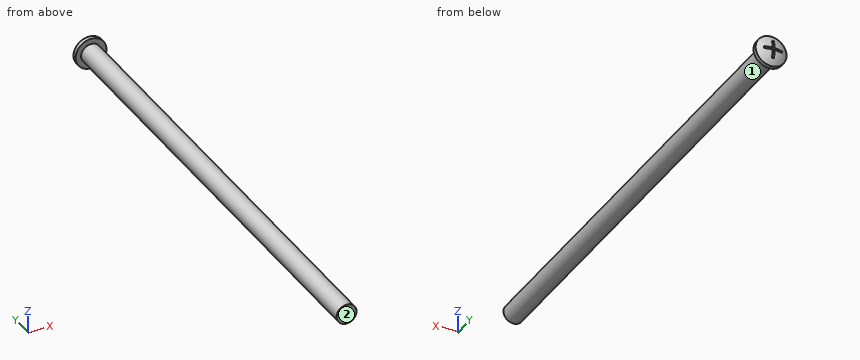
from build123d import *

# Parameters (mm, degrees)
CUT_EXTRUDE_2_DEPTH = 10


with BuildPart() as part:
    # 草图5 → 旋转1 (revolve)
    with BuildSketch(Plane.XY, mode=Mode.PRIVATE) as revolve_1_sk:
        with BuildLine():
            Line((0, -14), (-1, -14))
            Line((-1, -14), (-1, 35))
            Line((-1, 35), (-1.55, 35))
            Line((-1.55, 35), (-1.55, 35.411529967))
            add(Edge.make_bspline(
                [(-1.55, 35.411529967), (-0.860800082, 35.895988097), (0, 35.897418779)],
                knots=[0, 0, 0, 1, 1, 1], degree=2))
            Line((0, 35.897418779), (0, -14))
        make_face()
    revolve(revolve_1_sk.sketch.rotate(Axis((0, 0, 0), (0, 1, 0)), 270), axis=Axis((0, 0, 0), (0, 1, 0)))

    # 草图6 → 切除-拉伸2 (cut)
    with BuildSketch(Plane(origin=(0, 35.411529967, 0), x_dir=(-1, 0, 0), z_dir=(0, -1, 0))):
        Polygon((0.1, -0.1), (0.9, -0.1), (0.9, 0.1), (0.1, 0.1), (0.1, 0.9), (-0.1, 0.9), (-0.1, 0.1), (-0.9, 0.1), (-0.9, -0.1), (-0.1, -0.1), (-0.1, -0.9), (0.1, -0.9), align=None)
    extrude(amount=-CUT_EXTRUDE_2_DEPTH, mode=Mode.SUBTRACT)


solid = part.part
The listing builds one solid part. Answer for the finished solid, in the listing's coordinates (mm). Face numbers are marked on the shaded views. Round coordinates to 2 decimals unless told otherwise and drop trailing zeros. Write each loop counter-clockwise with the first axis right and the second up, starting at its lowest first coordinate (ties: lowest second). Pieces come first, ordered by that corner, then holes. Notation, with made-up numbers: M 26,42.25 L 40,42.25 A8 cw 40,50.25 Z; hole C 42,20 d7. An arc over 180 degrees is marked long. Write each question's results on one line, items separated by ' | '. Start each with the question number.
Item 1: The mould has two halves that part along Y. Classify the marked faces 1 and 2: +Y half, -Y half, draft (parallel to the pull), parting line (faces both ways), or undercut.
Item 2: Given pin 1 Ø0.5 at (y, z) = (35.5, 0.5) entering from +X; pin 2 Ø1.5 at (y, z) = (28, -1) entering from +X; pin 3 Ø0.5 at (x, y) = (0.5, 35.5) entering from -Z, each flat-ended and moving along its own axis, determine where each tip first touches the part or whether it passes through.
Item 3: Straight lines are drawn through the part: probe 1 along Z at (x, y) = (-0.05, 5); probe 2 along Y at (x, z) = (0.85, 0); probe 3 along Z at (x, y) = (-0.6, -11.5). For each, find the intervals that lie inside material, in ascending order.
Item 4: Find section A-A on y = 18.5. Write down the section's boundary in (x, z), and give its area (3 significant figures).
Answer block:
1) face 1: draft | face 2: -Y half
2) pin 1: stops at x = 1.53 | pin 2: stops at x = 0.97 | pin 3: stops at z = -1.53
3) probe 1: z = -1 to 1 | probe 2: y = -14 to 35.41 | probe 3: z = -0.8 to 0.8
4) outline: C 0,0 d2 | area: 3.14 mm²
